The model under review builds one solid part; all positions refer to its coordinate system, in mm. Round coordinates to 2 decimals unless told otherwise and drop trailing zeros. Write each loop counter-clockwise with the first axis right and the second up, starting at its lowest first coordinate (ties: lowest second). Pieces come first, ordered by that corner, then holes. Notation, with made-up numbers: (3.25, -19.75) - (47.25, -19.75) arc R7 ccw to (47.25, -7.75) - close; hole circle Ø2 at (65.5, -10.75). An arc over 180 degrees is marked (long way). Use one line per item in the form item = value.
from build123d import *

# Parameters (mm, degrees)
F0_W     = 25.4
F0_H     = 57.15
F0_R     = 1.5875
F1_DEPTH = 6.35
F2_R     = 6.35
F3_R     = 6.35


with BuildPart() as f1:
    # F0 (on Right) → F1 (new body)
    with BuildSketch(Plane.YZ):
        Rectangle(F0_W, F0_H)
        with Locations((0, -22.225)):
            Circle(F0_R, mode=Mode.SUBTRACT)
        with Locations((-6.35, 3.175)):
            Circle(F0_R, mode=Mode.SUBTRACT)
        with Locations((-6.35, 17.907)):
            Circle(F0_R, mode=Mode.SUBTRACT)
        with Locations((6.35, 3.175)):
            Circle(F0_R, mode=Mode.SUBTRACT)
        with Locations((6.35, 17.907)):
            Circle(F0_R, mode=Mode.SUBTRACT)
    extrude(amount=F1_DEPTH)

    # F2
    f2_edges = [f1.edges().sort_by_distance(p)[0] for p in [
        (3.175, -12.7, 28.575),
        (3.175, 12.7, 28.575),
    ]]
    fillet(f2_edges, radius=F2_R)

    # F3
    f3_edges = [f1.edges().sort_by_distance(p)[0] for p in [
        (3.175, -12.7, -28.575),
        (3.175, 12.7, -28.575),
    ]]
    fillet(f3_edges, radius=F3_R)


solid = f1.part
(1) Add section D-D on y = -9.5. Write out the cut boundary in (x, z).
Geometry results:
outline = (0, -27.74) - (6.35, -27.74) - (6.35, 27.74) - (0, 27.74) - close
(2) The part is to be moulded in two halves that separate along Y. For faces 1 (the cylindrical face through (3.219, 10.79, -26.764)), 2 (the cylindrical face through (3.219, -10.889, -26.665)), 3 (the cylindrical face through (3.13, 5.18, 4.25)), say which applies: +Y half, -Y half, draft (parallel to the pull), parting line (faces both ways), or undercut.
Geometry results:
face_1 = +Y half
face_2 = -Y half
face_3 = undercut
(3) To check wall thickness, follow L1, parallel to Z at x = 4.5, y = -6.35 (1 decimal); L2, parallel to Y at x = 3.25, z = 17; L3, parallel to Z at x = 1.75, y = -5.25 (3 decimals). State the ranges of each line that lie inside material, in increasing order.
Geometry results:
L1 = -28.6 to 1.6, 4.8 to 16.3, 19.5 to 28.6
L2 = -12.7 to -7.65, -5.05 to 5.05, 7.65 to 12.7
L3 = -28.575 to 2.03, 4.32 to 16.762, 19.052 to 28.575
(4) Add section B-B on x = 4.75. Count the separate pieces of the cut face and the enclosed holes in it, then the cut area to 3 significant figures.
Geometry results:
separate_pieces = 1
enclosed_holes = 5
area = 1,380 mm2
(5) Add section C-C on y = 9.75. Write out the cut boundary in (x, z).
Geometry results:
outline = (0, -27.59) - (6.35, -27.59) - (6.35, 27.59) - (0, 27.59) - close
